Check sheet for the modelled part. Datum: model origin and axes. Units: mm. A direction names the side the tool comes from. Give positions to 0.01 mm unless a question says otherwise; leave off trailing zeros. Order: outer loops, then holes, each group sorted by start corner. A loop starts at its lowest first (then second) coordinate and runs counter-clockwise, first axis right, second up. Notation, with made-up numbers: (16, 56.5) -> (51, 56.5) arc R25 ccw to (51, 75.5) -> close; hole circle Ø9 at (-25, 56). An arc over 180 degrees is marked (long way). Answer in a Markdown table with one row per item. Add a question column.
(1) Cross-section at C-C (y = 3). Record the cut outline in (x, z).
(2) Set-up check for faces 1 (the face through (5.76, -3.9, -3.58)), 2 (the face through (4.36, 6.68, 2.01)), 3 (the face through (3.723, -3.745, -0.57)): record each of +Z, -Z, +X, -X, +Y, -Y from which the full face is reachable in a straight line by a thin tool's end or side.
(3) Cross-section at B-B (z = -9). Record the cut outline in (x, y).
(4) Go/stop test with flat-tipped pins: pin 1 (4 mm diameter, centred on x = 3, y = 7.5, fed in from -Z); pin 2 (1 mm diameter, centred on y = -2.5, z = -8, fed in from -X); pin 3 (6 mm diameter, centred on y = -0.5, z = 0, fed in from +X); pin 4 (1.9 mm diameter, centred on x = -1, y = 0, fed in from -Z). Record where each tip stops, or that it passes through.
(5) Cross-section at A-A (y = 0.5). Record the cut outline in (x, z), then the cut area to 3 significant figures.
(6) Thickness scan on L1, parallel to Y at x = 0, z = 0.25; L2, parallel to Z at x = 0.75, y = -2; L3, parallel to Z at x = -3, y = 3.5. Record the ranges inside material, lowest first. Write a range as [from, to].
(7) Release check for a two-part mould opening along Z. For faces 4 (the face through (3.974, -3.871, -2.581)), 5 (the face through (6.28, -5.31, -3.9)), 6 (the face through (5.48, -4.81, -6.78)) record: released by +Z, released by -Z, zero draft, split by the parting line, or undercut.
Autodesk Inventor part; units mm, degrees
ref_plane "YZ Plane" through (0, 0, 0) normal (1, 0, 0) x (0, 1, 0)
ref_plane "XZ Plane" through (0, 0, 0) normal (0, 1, 0) x (-1, 0, 0)
ref_plane "XY Plane" through (0, 0, 0) normal (0, 0, 1) x (1, 0, 0)
sketch "Skizze1" plane through (0, 0, 0) normal (0, 0, 1) x (1, 0, 0)
  circle A0 centre (0, 0) radius 0.5718 construction
  circle A1 centre (0, 0) radius 1.1
  line L0 (-3.4324, -5.4831) -> (-0.3524, -0.608)
  line L1 (12.1628, 19.8522) -> (1.5943, 2.5967)
  line L2 (0, 0) -> (-2.7013, -4.3259)
  line L3 (0, 0) -> (2.6665, 4.3474)
  line L4 (0, 0) -> (4.3474, -2.6665)
  line L5 (1.6594, -7.0489) -> (-6.9075, -1.6993)
  line L6 (-6.9075, -1.6993) -> (-1.5201, 6.9282)
  line L7 (-1.5201, 6.9282) -> (7.0468, 1.5787)
  line L8 (7.0468, 1.5787) -> (1.6594, -7.0489)
  dimension "d0" = 2.2
  dimension "d1" = 5.1
  dimension "d2" = 5.1
  dimension "d3" = 5.1
  dimension "d4" = 10.1
extrude "Extrusion1" add sketch "Skizze1" along normal blind 3 contours A1 L3 L1 L7 L8 L5 L0 | A1 L2 L5 L6 L7 L1 L3 | A1 L0 L2
sketch "Skizze2" plane through (0, 0, 0) normal (0, 0, -1) x (-1, 0, 0)
  circle A0 centre (0, 0) radius 1.1
  line L0 (-1.6594, -7.0489) -> (6.9075, -1.6993)
  line L1 (6.9075, -1.6993) -> (1.5201, 6.9282)
  line L2 (1.5201, 6.9282) -> (-7.0468, 1.5787)
  line L3 (-7.0468, 1.5787) -> (-1.6594, -7.0489)
  circle A1 centre (0, 0) radius 1.1
  circle A2 centre (0.0269, 0) radius 2.5
  dimension "d7" = 5
extrude "Extrusion2" cut sketch "Skizze2" against normal blind 1 contours L3 L2 L1 L0
sketch "Skizze3" plane through (0, 0, 3) normal (0, 0, 1) x (1, 0, 0)
  circle A0 centre (0, 0) radius 1.1
  line L0 (-6.9075, -1.6993) -> (1.6594, -7.0489)
  line L1 (1.6594, -7.0489) -> (7.0468, 1.5787)
  line L2 (7.0468, 1.5787) -> (-1.5201, 6.9282)
  line L3 (-1.5201, 6.9282) -> (-6.9075, -1.6993)
  line L4 (-2.6241, -4.3741) -> (-1.1, -1.79)
  line L5 (-6.9075, -1.6993) -> (1.6594, -7.0489)
  line L6 (1.6594, -7.0489) -> (3.2354, -4.5251)
  line L7 (3.2354, -4.5251) -> (-5.3316, 0.8245)
  line L8 (-5.3316, 0.8245) -> (-6.9075, -1.6993)
  dimension "d10" = 3
extrude "Extrusion3" cut sketch "Skizze3" against normal through all contours L3 L7 L4 L0 | L4 L7 L1 L0
sketch "Skizze4" plane through (0, 0, 3) normal (0, 0, 1) x (1, 0, 0)
  line L0 (-5.3316, 0.8245) -> (3.2354, -4.5251)
  line L1 (3.2354, -4.5251) -> (7.0468, 1.5787)
  line L2 (7.0468, 1.5787) -> (-1.5201, 6.9282)
  line L3 (-1.5201, 6.9282) -> (-5.3316, 0.8245)
  circle A0 centre (0, 0) radius 1.1
  line L4 (-5.3316, 0.8245) -> (3.2354, -4.5251)
  line L5 (-5.3316, 0.8245) -> (3.2354, -4.5251)
  line L6 (3.2354, -4.5251) -> (8.5849, 4.0418)
  line L7 (8.5849, 4.0418) -> (0.018, 9.3914)
  line L8 (0.018, 9.3914) -> (-5.3316, 0.8245)
  dimension "d13" = 10.1
extrude "Extrusion4" add sketch "Skizze4" against normal up to surface (2 mm away) contours L8 L7 L6 L2
sketch "Skizze5" plane through (0, 0, 3) normal (0, 0, 1) x (1, 0, 0)
  line L0 (4.2881, -6.9427) -> (6.1322, -4.0444)
  line L1 (5.7598, -3.8294) -> (4.7032, -3.2194)
  line L2 (-5.3316, 0.8245) -> (3.2354, -4.5251)
  line L3 (3.2354, -4.5251) -> (8.5849, 4.0418)
  line L4 (8.5849, 4.0418) -> (0.018, 9.3914)
  line L5 (0.018, 9.3914) -> (-5.3316, 0.8245)
  circle A0 centre (0, 0) radius 1.1
  line L6 (3.2354, -4.5251) -> (8.5849, 4.0418)
  line L7 (3.2354, -4.5251) -> (4.2236, -2.9426)
  line L8 (4.2236, -2.9426) -> (7.6164, -5.0612)
  line L9 (7.6164, -5.0612) -> (6.6282, -6.6437)
  line L10 (6.6282, -6.6437) -> (3.2354, -4.5251)
  dimension "d16" = 4
extrude "Extrusion5" add sketch "Skizze5" against normal blind 14 contours L10 L3 L8 L0 | L0 L8 L9 L10
sketch "Skizze6" plane through (7.6164, -5.0612, 3) normal (0.5296614, 0.8482092, 0) x (0.8482092, -0.5296614, 0)
  line L0 (-1.7975, 12.28) -> (-2.2192, 15.496)
  line L1 (-1.9046, 10.7265) -> (-1.9053, 12.2728)
  line L2 (-1.9046, 10.7265) -> (-2.6926, 7.736)
  line L3 (-2.2272, 9.066) -> (-3.4465, 6.126)
  line L4 (-4.252, 5.184) -> (-3.4465, 6.126)
  line L5 (-4, 2) -> (-4, 14)
  arc A0 (-4, 5.4787) -> (-2.0084, 13.888) centre (-13.8052, 12.2414) ccw construction
  arc A1 (-3.4465, 5.9662) -> (-1.8224, 14) centre (-13.8052, 12.2414) ccw
  line L6 (-4, 14) -> (0, 14)
  line L7 (-1.8224, 14) -> (-4, 14)
  line L8 (-4, 14) -> (-4, 5.1324)
  line L9 (-1.9018, 5.1324) -> (-1.8224, 5.1324)
  line L10 (-3.4465, 5.9662) -> (-4, 5.184)
  point P0 (-9.141, 3)
extrude "Extrusion6" cut sketch "Skizze6" against normal through all
sketch "Skizze7" plane through (6.6282, -6.6437, 3) normal (0.8482092, -0.5296614, 0) x (0, 0, -1)
  line L0 (0, 0) -> (0, 1.8657)
  line L1 (0, 0) -> (14, 0)
  line L2 (14, 1.8657) -> (14, 0)
  line L3 (0, 1.8657) -> (14, 1.8657)
  point P0 (3, 2.1246)
extrude "Extrusion7" cut sketch "Skizze7" against normal blind 1
sketch "Skizze8" plane through (0, 0, 3) normal (0, 0, 1) x (1, 0, 0)
  circle A0 centre (0, 0) radius 1.1
  line L0 (5.78, -6.1141) -> (6.7682, -4.5315)
  line L1 (6.7682, -4.5315) -> (4.2236, -2.9426)
  line L2 (4.2236, -2.9426) -> (8.5849, 4.0418)
  line L3 (8.5849, 4.0418) -> (0.018, 9.3914)
  line L4 (0.018, 9.3914) -> (-5.3316, 0.8245)
  line L5 (-5.3316, 0.8245) -> (5.78, -6.1141)
  line L6 (6.7682, -4.5315) -> (8.5849, 4.0418)
extrude "Extrusion8" add sketch "Skizze8" against normal up to surface (2 mm away) contours L1 L2 L6
properties part number "thumb_base_plate" material "Nylon 6/6"
Answer below:
| question | item | result |
|---|---|---|
| 1 | outline | (-3.97, 1) -> (8.36, 1) -> (8.36, 3) -> (-3.97, 3) -> close |
| 2 | face 1 | -Z, +X, +Y |
| 2 | face 2 | +Z, -Z, +X, +Y |
| 2 | face 3 | -Z, -X, +Y |
| 3 | outline | (5.19, -5.75) -> (5.78, -6.11) -> (6.77, -4.53) -> (6.18, -4.16) -> close |
| 4 | pin 1 | stops at z = 1 |
| 4 | pin 2 | passes through |
| 4 | pin 3 | stops at x = 8.22 |
| 4 | pin 4 | stops at z = 0 |
| 5 | outline | (-4.81, 1) -> (-2.48, 1) -> (-2.48, 0) -> (-0.98, 0) -> (-0.98, 3) -> (-4.81, 3) -> close; (0.98, 0) -> (2.42, 0) -> (2.42, 1) -> (7.83, 1) -> (7.83, 3) -> (0.98, 3) -> close |
| 5 | area | 24.3 mm² |
| 6 | L1 | y = [-2.5, -1.1], [1.1, 2.5] |
| 6 | L2 | z = [0, 3] |
| 6 | L3 | z = [1, 3] |
| 7 | face 4 | released by -Z |
| 7 | face 5 | zero draft |
| 7 | face 6 | undercut |
